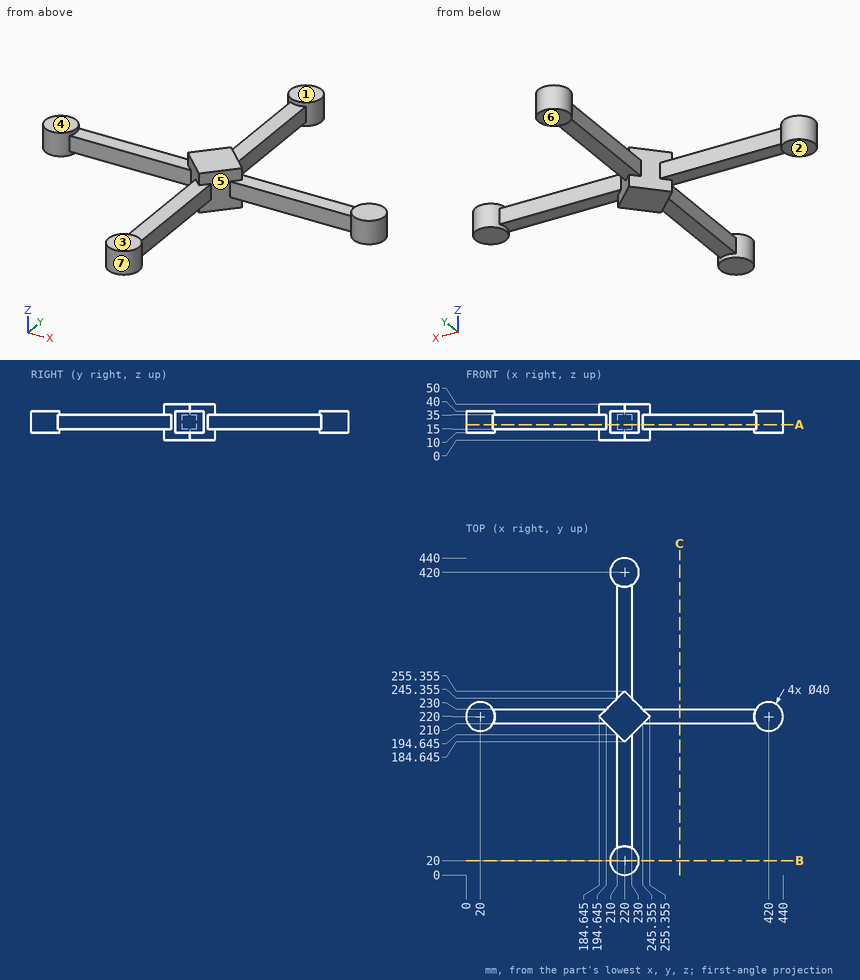
Print and shaded views of the part. All mm, measured from the part's lowest x, y and z. A direction names the side the tool comes from. Coordinates: 2 decimals unless noted, no trailing zeros. Order: outer loops, then holes, each group sorted by start corner. A loop starts at its lowest first (then second) coordinate and runs counter-clockwise, first axis right, second up. Notation, with made-up numbers: M 54,80.25 L 89,80.25 A21 cw 89,100.25 Z; hole C 40,45 d1. An arc over 180 degrees is marked long. Answer as CSV lines item,"result".
1) Cut at B-B (y = 20). List the corners of the cut face in (x, z), then the cut area to 3 significant figures.
Verdict:
outline,"M 200,10 L 240,10 L 240,40 L 200,40 Z"
area,"1,200 mm2"
2) Flat gauge pins, fed straight in: P1, Ø6, axis at x = 261, y = 232.5, coming from the +Z side; P2, Ø10, axis at x = 220.5, y = 150, coming from the -Z side; P3, Ø20, axis at x = 221, y = 410, coming from the +Z side. Where does each tip first touch, or does it go through?
Verdict:
P1,"z = 35"
P2,"z = 15"
P3,"z = 40"
3) 3-axis set-ups, long thin cutter, end or side, ignore diameter. For the marked faces 1, 2, 3 and 4: which of +Z, -Z, +X, -X, +Y, -Y reach the whole face in a straight line?
Verdict:
face 1,"+Z, +X, -X, +Y"
face 2,"-Z, -X, +Y, -Y"
face 3,"+Z, +X, -X, -Y"
face 4,"+Z, -X, +Y, -Y"
4) Cut at C-C (x = 296.5). List the corners of the cut face in (y, z).
Verdict:
outline,"M 210,15 L 230,15 L 230,35 L 210,35 Z"
5) Mould opens along X. For the marked faces 5, 6 and 7 say: released by +X, released by -X, zero draft, split by the parting line, or undercut.
Verdict:
face 5,"undercut"
face 6,"zero draft"
face 7,"split by the parting line"
6) Drill centre lines: L1, parallel to Z at x = 122, y = 219.5; L2, parallel to X at y = 390.5, z = 18. Where is each one in solid material? Low to high. Write a range as from..to.
Verdict:
L1,"15..35"
L2,"210..230"
7) Cut at A-A (z = 21.5). List the corners of the cut face in (x, y) (1 decimal).
Verdict:
outline,"M 37.3,210 L 194.6,210 L 210,194.6 L 210,37.3 A20 ccw long 230,37.3 L 230,194.6 L 245.4,210 L 402.7,210 A20 ccw long 402.7,230 L 245.4,230 L 230,245.4 L 230,402.7 A20 ccw long 210,402.7 L 210,245.4 L 194.6,230 L 37.3,230 A20 ccw long Z"
